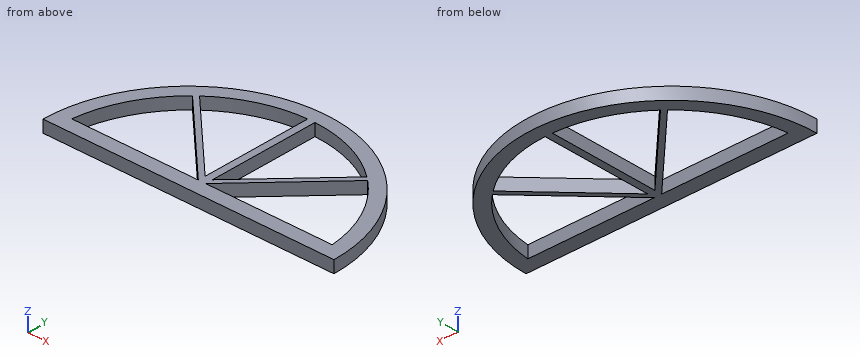
```python
from build123d import *

# Parameters (mm, degrees)
F1_DEPTH = 25


with BuildPart() as f1:
    # F0 (on Top) → F1 (new body)
    with BuildSketch(Plane.XY):
        with BuildLine():
            ThreePointArc((534.253372, -30), (234.253372, 270), (-65.746628, -30))
            Line((-65.746628, -30), (534.253372, -30))
        make_face()
        with BuildLine():
            Line((226.753372, 0), (-34.335003, 0))
            ThreePointArc((-34.335003, 0), (-6.452084, 94.741433), (53.635165, 173.118207))
            Line((53.635165, 173.118207), (226.753372, 0))
        make_face(mode=Mode.SUBTRACT)
        with BuildLine():
            ThreePointArc((414.871579, 173.118207), (474.958829, 94.741433), (502.841748, 0))
            Line((502.841748, 0), (241.753372, 0))
            Line((241.753372, 0), (414.871579, 173.118207))
        make_face(mode=Mode.SUBTRACT)
        with BuildLine():
            Line((226.753372, 242.322557), (226.753372, 15))
            Line((226.753372, 15), (61.678279, 180.075094))
            ThreePointArc((61.678279, 180.075094), (138.988234, 225.061962), (226.753372, 242.322557))
        make_face(mode=Mode.SUBTRACT)
        with BuildLine():
            Line((406.828466, 180.075094), (241.753372, 15))
            Line((241.753372, 15), (241.753372, 242.322557))
            ThreePointArc((241.753372, 242.322557), (329.51851, 225.061962), (406.828466, 180.075094))
        make_face(mode=Mode.SUBTRACT)
    extrude(amount=F1_DEPTH)


solid = f1.part
```
The listing builds one solid part. Answer for the finished solid, in the listing's coordinates (mm). Round coordinates to 2 decimals unless told otherwise and drop trailing zeros. Loops run counter-clockwise (first coordinate to the right, second up) from the corner with the lowest first, then second, coordinate; pieces in that order, holes last. Notation, with made-up numbers: (-7.75, 44.25) - (14.25, 44.25) arc R9 ccw to (14.25, 60.25) - close; hole circle Ø6 at (52, 52). An arc over 180 degrees is marked (long way). Use one line per item in the form item = value. Start each with the question number.
1. Consider line 1 (X direction, y = 174, z = 15.5); line 2 (X direction, y = 16.5, z = 16.5); line 3 (Y direction, x = 333.5, z = 17.5). Determine where each line is inside the solid, lowest interval first. Write a range as [from, to].
2. The part is cut by section C-C on y = 205. Determine the outline of the cut face in (x, z).
3. Given pin 1 Ø1 at (x, z) = (343, 11.5) entering from +Y; pin 2 Ø6 at (x, z) = (456.5, 5) entering from +Y; pin 3 Ø1.5 at (y, z) = (106.5, 7.5) entering from +X, each flat-ended and moving along its own axis, determine where each tip first touches the part or whether it passes through.
4. The part is cut by section B-B on x = 323.5. Determine the outline of the cut face in (y, z).
5. The part is cut by section A-A on z = 12.5. Determine the outline of the cut face in (x, y) (3 decimals), then the cut area to 3 significant figures.
6. The part is cut by section D-D on x = 6.5. Determine the outline of the cut face in (y, z), then the cut area to 3 significant figures.
Geometry check:
q1.line_1 = [14.29, 67.75], [226.75, 241.75], [400.75, 454.22]
q1.line_2 = [-62.12, -32.13], [210.25, 225.25], [226.75, 241.75], [243.25, 258.25], [500.63, 530.63]
q1.line_3 = [-30, 0], [91.75, 106.75], [223.52, 253.11]
q2.outline = (47.77, 0) - (97.1, 0) - (97.1, 25) - (47.77, 25) - close; (226.75, 0) - (241.75, 0) - (241.75, 25) - (226.75, 25) - close; (371.4, 0) - (420.73, 0) - (420.73, 25) - (371.4, 25) - close
q3.pin_1 = 249.79
q3.pin_2 = 174.77
q3.pin_3 = 501.78
q4.outline = (-30, 0) - (0, 0) - (0, 25) - (-30, 25) - close; (81.75, 0) - (96.75, 0) - (96.75, 25) - (81.75, 25) - close; (227.25, 0) - (256.42, 0) - (256.42, 25) - (227.25, 25) - close
q5.outline = (-65.747, -30) - (534.253, -30) arc R300 ccw to start; hole (-34.335, 0) - (226.753, 0) - (53.635, 173.118) arc R270 ccw to start; hole (61.678, 180.075) - (226.753, 15) - (226.753, 242.323) arc R270 ccw to start; hole (241.753, 0) - (502.842, 0) arc R270 ccw to (414.872, 173.118) - close; hole (241.753, 15) - (406.828, 180.075) arc R270 ccw to (241.753, 242.323) - close
q5.area = 50,400 mm^2
q6.outline = (-30, 0) - (0, 0) - (0, 25) - (-30, 25) - close; (117.44, 0) - (165.26, 0) - (165.26, 25) - (117.44, 25) - close
q6.area = 1,950 mm^2
